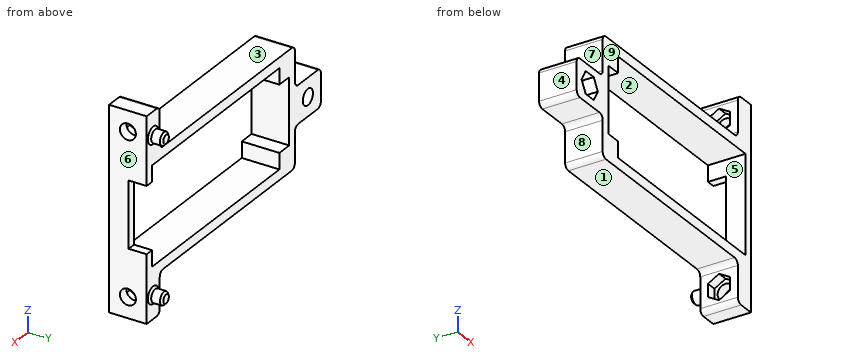
```python
from build123d import *

# Parameters (mm, degrees)
CROQUIS1_R              = 1.55
SALIENTE_EXTRUIR1_DEPTH = 7.3
CROQUIS5_W              = 12.8
CROQUIS5_H              = 3.5
CORTAR_EXTRUIR4_DEPTH   = 1.65
CORTAR_EXTRUIR5_DEPTH   = 5
CROQUIS6_W              = 7.965212315
CROQUIS6_H              = 7.3
CROQUIS6_R              = 1.55
SALIENTE_EXTRUIR2_DEPTH = 4
CORTAR_EXTRUIR6_DEPTH   = 2
REDONDEO1_R             = 1
CROQUIS8_R              = 1.25
SALIENTE_EXTRUIR3_DEPTH = 2.5
CHAFL_N1_SIZE           = 0.4


with BuildPart() as part:
    # Croquis1 → Saliente-Extruir1 (new body)
    with BuildSketch(Plane(origin=(0, 0, 0), x_dir=(1, 0, 0), z_dir=(0, 1, 0))):
        Polygon((-24.25, 11.5), (-24.25, 3.65), (-32.215212315, 3.65), (-32.215212315, -3.65), (-24.25, -3.65), (-24.25, -11.5), (21.15, -11.5), (21.15, 11.5), align=None)
        with Locations((-28.232606158, 0)):
            Circle(CROQUIS1_R, mode=Mode.SUBTRACT)
        Polygon((-19.5, 9.5), (19.5, 9.5), (19.5, 6.4), (19.5, -6.4), (19.5, -9.5), (-19.5, -9.5), (-19.5, -6.4), (-22.5, -6.4), (-22.5, 6.4), (-19.5, 6.4), align=None, mode=Mode.SUBTRACT)
    extrude(amount=SALIENTE_EXTRUIR1_DEPTH)

    # Croquis5 → Cortar-Extruir4 (cut)
    with BuildSketch(Plane(origin=(21.15, 0, 0), x_dir=(0, 0, -1), z_dir=(1, 0, 0))):
        with Locations((0, 5.55)):
            Rectangle(CROQUIS5_W, CROQUIS5_H)
    extrude(amount=-CORTAR_EXTRUIR4_DEPTH, mode=Mode.SUBTRACT)

    # Croquis4 → Cortar-Extruir5 (cut)
    with BuildSketch(Plane.XZ):
        Polygon((-26.991303079, 2.15), (-25.75, 0), (-26.991303079, -2.15), (-29.473909236, -2.15), (-30.715212315, 0), (-29.473909236, 2.15), align=None)
    extrude(amount=-CORTAR_EXTRUIR5_DEPTH, mode=Mode.SUBTRACT)

    # Croquis6 → Saliente-Extruir2 (add)
    with BuildSketch(Plane(origin=(21.15, 0, 0), x_dir=(0, 0, -1), z_dir=(1, 0, 0))):
        with Locations((15.482606158, 3.65)):
            Rectangle(CROQUIS6_W, CROQUIS6_H)
        with Locations((15.482606158, 3.65)):
            Circle(CROQUIS6_R, mode=Mode.SUBTRACT)
        with Locations((-15.482606158, 3.65)):
            Rectangle(CROQUIS6_W, CROQUIS6_H)
        with Locations((-15.482606158, 3.65)):
            Circle(CROQUIS6_R, mode=Mode.SUBTRACT)
    extrude(amount=-SALIENTE_EXTRUIR2_DEPTH)

    # Croquis7 → Cortar-Extruir6 (cut)
    with BuildSketch(Plane.ZY.offset(-17.15)):
        Polygon((-17.965212315, 3.65), (-16.723909236, 5.8), (-14.241303079, 5.8), (-13, 3.65), (-14.241303079, 1.5), (-16.723909236, 1.5), align=None)
        Polygon((16.723909236, 1.5), (17.965212315, 3.65), (16.723909236, 5.8), (14.241303079, 5.8), (13, 3.65), (14.241303079, 1.5), align=None)
    extrude(amount=-CORTAR_EXTRUIR6_DEPTH, mode=Mode.SUBTRACT)

    # Redondeo1
    redondeo1_edges = [part.edges().sort_by_distance(p)[0] for p in [
        (17.15, 3.65, 11.5),
        (17.15, 3.65, 19.465212315),
        (-24.25, 3.65, 11.5),
        (-24.25, 3.65, 3.65),
        (-32.215212315, 3.65, 3.65),
        (-32.215212315, 3.65, -3.65),
        (-24.25, 3.65, -3.65),
        (-24.25, 3.65, -11.5),
        (17.15, 3.65, -19.465212315),
        (17.15, 3.65, -11.5),
    ]]
    fillet(redondeo1_edges, radius=REDONDEO1_R)

    # Croquis8 → Saliente-Extruir3 (add)
    with BuildSketch(Plane(origin=(0, 7.3, 0), x_dir=(1, 0, 0), z_dir=(0, 1, 0))):
        with Locations((19.15, -14.965212315)):
            Circle(CROQUIS8_R)
        with Locations((19.15, 14.965212315)):
            Circle(CROQUIS8_R)
    extrude(amount=SALIENTE_EXTRUIR3_DEPTH)

    # Chaflán1
    chafl_n1_edges = [part.edges().sort_by_distance(p)[0] for p in [
        (17.9, 7.3, 14.965212315),
        (17.9, 9.8, 14.965212315),
        (17.9, 7.3, -14.965212315),
        (17.9, 9.8, -14.965212315),
    ]]
    chamfer(chafl_n1_edges, length=CHAFL_N1_SIZE)


solid = part.part
```
Check sheet for the modelled part. Datum: model origin and axes. Units: mm. Face numbers are marked on the shaded views. A direction names the side the tool comes from. Round coordinates to 2 decimals unless told otherwise and drop trailing zeros. Write each loop counter-clockwise with the first axis right and the second up, starting at its lowest first coordinate (ties: lowest second). Pieces come first, ordered by that corner, then holes. Notation, with made-up numbers: M 33,46.5 L 74,46.5 A18 cw 74,65.5 Z; hole C -12.75,40 d8. An arc over 180 degrees is marked long. Write item = value, one per line. Start each with the question number.
1. Tool access check on the marked faces 5, 6, 7, 8 and 9. Record the directions out of +Z, -Z, +X, -X, +Y, -Y that give a thin tool (end or side, any length) a straight path to the whole face; none if there is none.
2. Scan lines: line 1 (Z direction, x = -4, y = 7.25); line 2 (Z direction, x = -21.5, y = 7); line 3 (Z direction, x = 18, y = 3). Record each from-to range of solid material in increasing order. Write a range as [from, to].
3. Section check B-B, the plane x = -1. Record the cut outline in (y, z), then the cut area to 3 significant figures.
4. Release check for a two-part mould opening along Z. For the marked faces 1, 2, 3 and 4 record: pulls with the +Z half, pulls with the -Z half, needs draft (parallel to the pull), parting line crosses it, or undercut.
5. Section check A-A, the plane z = 7. Record the cut outline in (x, y).
6. Gauge pin test, flat ends, axial feed: pin 1 (5 mm diameter, centred on x = -28, y = 3, fed in from +Z); pin 2 (3.5 mm diameter, centred on x = -8.5, y = 3, fed in from +Z); pin 3 (1.2 mm diameter, centred on x = -28.5, y = 1.5, fed in from -Z). Record the tip position at first contact, or that the pin passes through.
Results found:
q1.face_5 = +Y, -Y
q1.face_6 = +Z, -Z, +X, +Y, -Y
q1.face_7 = +Z, -X, +Y, -Y
q1.face_8 = -Z, -X, +Y, -Y
q1.face_9 = +Z, -Z, +X, -X, -Y
q2.line_1 = [-11.5, -9.5], [9.5, 11.5]
q2.line_2 = [-11.5, -6.4], [6.4, 11.5]
q2.line_3 = [-19.45, -17.59], [-13.38, -9.5], [9.5, 13.38], [17.59, 19.45]
q3.outline = M 0,-11.5 L 7.3,-11.5 L 7.3,-9.5 L 0,-9.5 Z; M 0,9.5 L 7.3,9.5 L 7.3,11.5 L 0,11.5 Z
q3.area = 29.2 mm^2
q4.face_1 = pulls with the -Z half
q4.face_2 = undercut
q4.face_3 = pulls with the +Z half
q4.face_4 = needs draft
q5.outline = M -24.25,0 L -19.5,0 L -19.5,7.3 L -24.25,7.3 Z; M 19.5,0 L 21.15,0 L 21.15,7.3 L 19.5,7.3 Z
q6.pin_1 = 3.65
q6.pin_2 = 11.5
q6.pin_3 = -3.65
